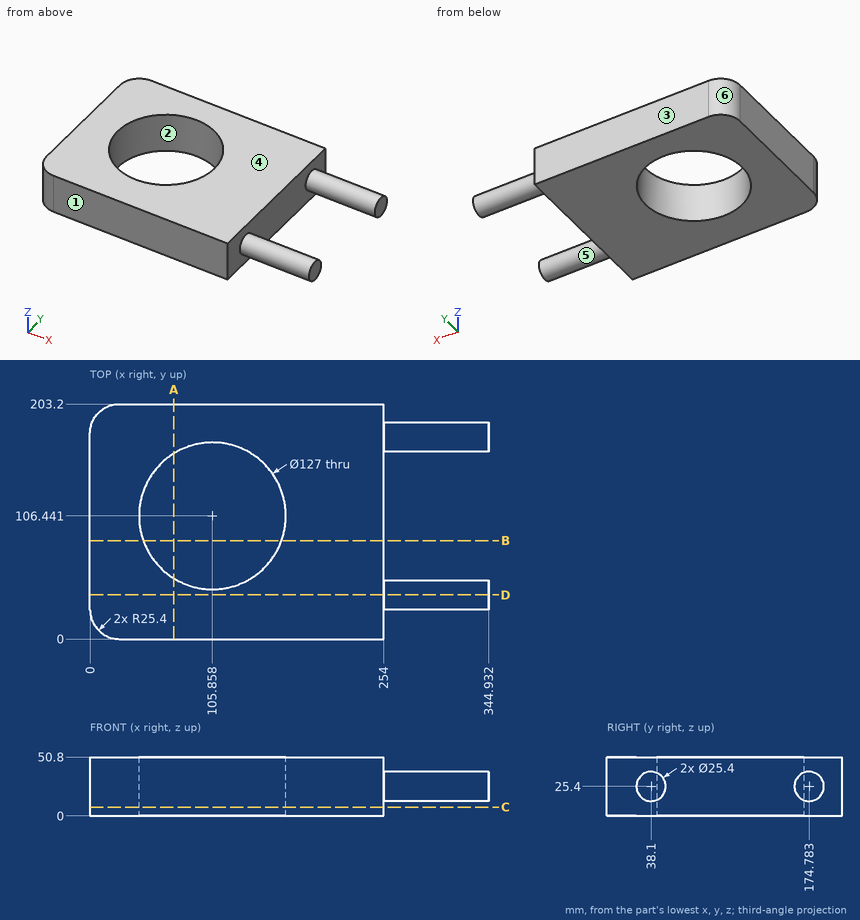
Design review of the part shown in the three views and the two pictorial views. Dimensions are in mm from the part's minimum x, y and z. A direction names the side the tool comes from. Round coordinates to 2 decimals unless told otherwise and drop trailing zeros. Write each loop counter-clockwise with the first axis right and the second up, starting at its lowest first coordinate (ties: lowest second). Pieces come first, ordered by that corner, then holes.
1) Mouldability with a two-part tool opening along Y and no side actions: class the marked faces 1, 2, 3 and 4 as +Y half, -Y half, draft (parallel to the pull), parting line (faces both ways), or undercut.
Answer below:
face 1: -Y half
face 2: undercut
face 3: +Y half
face 4: draft
2) Take a section at D-D on y = 38.1. Give the boundary of the cut face in (x, z), then the cut area to 3 significant figures.
Answer below:
outline: (0, 0) - (254, 0) - (254, 12.7) - (344.93, 12.7) - (344.93, 38.1) - (254, 38.1) - (254, 50.8) - (0, 50.8) - close
area: 15,200 mm2
3) Take a section at C-C on z = 7.5. Give the boundary of the cut face in (x, y), then the cut area to 3 significant figures.
Answer below:
outline: (0, 25.4) arc R25.4 ccw to (25.4, 0) - (254, 0) - (254, 203.2) - (25.4, 203.2) arc R25.4 ccw to (0, 177.8) - close; hole circle Ø127 at (105.86, 106.44)
area: 38,700 mm2
4) Machinability: for the marked faces 5 and 6, which of the approach directions +Z, -Z, +X, -X, +Y, -Y give a long, thin tool a straight path to every point of the face, cutting with its end or side? Answer none if there is none.
Answer below:
face 5: +X
face 6: +Z, -Z, -X, +Y
5) Take a section at B-B on y = 85. Give the boundary of the cut face in (x, z), then the cut area to 3 significant figures.
Answer below:
outline: (0, 0) - (46.09, 0) - (46.09, 50.8) - (0, 50.8) - close; (165.63, 0) - (254, 0) - (254, 50.8) - (165.63, 50.8) - close
area: 6,830 mm2
6) For line 1 along Y through (x, z) = (108, 11) (1 decimal); line 2 along X through (y, z) = (37.5, 39.5); line 3 along Y through (x, z) = (136.5, 27.5) (1 decimal), list the stretches that pass through material, from the lowest coordinate up.
Answer below:
line 1: y = 0 to 43, 169.9 to 203.2
line 2: x = 0 to 254
line 3: y = 0 to 50.8, 162.1 to 203.2
7) Take a section at A-A on x = 72.5. Give the boundary of the cut face in (y, z).
Answer below:
outline: (0, 0) - (52.41, 0) - (52.41, 50.8) - (0, 50.8) - close; (160.47, 0) - (203.2, 0) - (203.2, 50.8) - (160.47, 50.8) - close
